Can you work these out from the model? Positions are in its coordinate system, mm. Face numbers are marked on the shaded views. A direction names the side the tool comes from. Coordinates: 2 decimals unless noted, no trailing zeros. Order: outer loops, then holes, each group sorted by start corner. A loop starts at its lowest first (then second) coordinate and runs counter-clockwise, first axis right, second up. Notation, with made-up numbers: (34, -27.5) -> (92, -27.5) arc R18 ccw to (92, -9.5) -> close; hole circle Ø9 at (38.5, 45.5). An arc over 180 degrees is marked (long way). Answer in a Markdown table with one row per item.
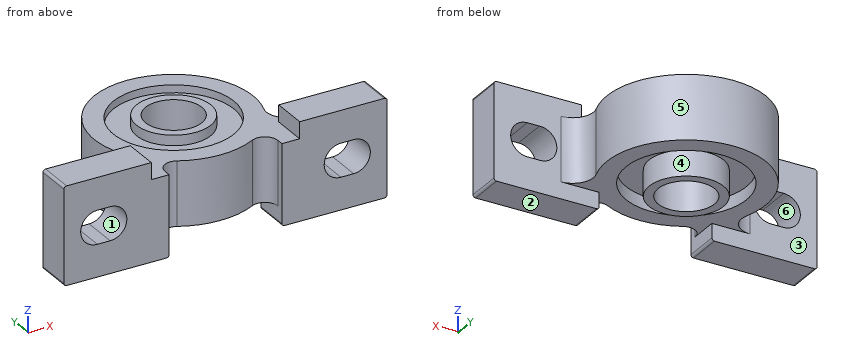
```python
from build123d import *

# Parameters (mm, degrees)
SKETCH_8_R          = 14.5
SKETCH_8_R_2        = 11
EXTRUDE_1_DEPTH     = 31
SKETCH_10_R         = 23.5
SKETCH_10_R_2       = 14.5
EXTRUDE_2_DEPTH     = 17
EXTRUDE_START       = -5
SKETCH_11_R         = 31
SKETCH_11_R_2       = 23.5
EXTRUDE_3_DEPTH     = 25
SKETCH_13_W         = 41
SKETCH_13_H         = 38
EXTRUDE_4_DEPTH     = 14
FILLET_1_R          = 8
FILLET_2_R          = 5
FILLET_3_R          = 5
FILLET_4_R          = 8
FILLET_5_R          = 1
FILLET_6_R          = 1
SKETCH_14_W         = 12.689774382
SKETCH_14_H         = 9.496761799
CUT_EXTRUDE_5_DEPTH = 130.435312029


with BuildPart() as part:
    # Эскиз8 → Вытянуть1 (new body)
    with BuildSketch(Plane.XY):
        with Locations((50, -1.5)):
            Circle(SKETCH_8_R)
        with Locations((50, -1.5)):
            Circle(SKETCH_8_R_2, mode=Mode.SUBTRACT)
    extrude(amount=EXTRUDE_1_DEPTH)

    # Эскиз10 → Вытянуть2 (add)
    with BuildSketch(Plane.XY.offset(10)):
        with Locations((50, -1.5)):
            Circle(SKETCH_10_R)
        with Locations((50, -1.5)):
            Circle(SKETCH_10_R_2, mode=Mode.SUBTRACT)
    extrude(amount=EXTRUDE_2_DEPTH)

    # Эскиз11 → Вытянуть3 (add)
    with BuildSketch(Plane.XY.offset(10).offset(EXTRUDE_START)):
        with Locations((50, -1.5)):
            Circle(SKETCH_11_R)
        with Locations((50, -1.5)):
            Circle(SKETCH_11_R_2, mode=Mode.SUBTRACT)
    extrude(amount=EXTRUDE_3_DEPTH)

    # Эскиз13 → Вытянуть4 (add)
    # profile 1 of 2: a face of its own
    with BuildSketch(Plane(origin=(0, -36, 0), x_dir=(-1, 0, 0), z_dir=(0, 1, 0))):
        with Locations((-7.5, 17.5)):
            Rectangle(SKETCH_13_W, SKETCH_13_H)
        with BuildLine():
            Line((-4.740103958, 23.994802079), (0, 24))
            ThreePointArc((0, 24), (6.5, 17.5), (0, 11))
            Line((0, 11), (-5, 11))
            ThreePointArc((-5, 11), (-11.49870039, 17.629974008), (-4.740103958, 23.994802079))
        make_face(mode=Mode.SUBTRACT)
    # profile 2 of 2: a face of its own
    with BuildSketch(Plane(origin=(0, -36, 0), x_dir=(-1, 0, 0), z_dir=(0, 1, 0))):
        with Locations((-92.5, 17.5)):
            Rectangle(SKETCH_13_W, SKETCH_13_H)
        with BuildLine():
            Line((-95, 11), (-100, 11))
            ThreePointArc((-100, 11), (-106.5, 17.5), (-100, 24))
            Line((-100, 24), (-95.259896042, 23.994802079))
            ThreePointArc((-95.259896042, 23.994802079), (-88.50129961, 17.629974008), (-95, 11))
        make_face(mode=Mode.SUBTRACT)
    extrude(amount=EXTRUDE_4_DEPTH)

    # Скругление1
    fillet_1_edges = [part.edges().sort_by_distance(p)[0] for p in [
        (26.745968092, -22, 17.5),
    ]]
    fillet(fillet_1_edges, radius=FILLET_1_R)

    # Скругление2
    fillet_2_edges = [part.edges().sort_by_distance(p)[0] for p in [
        (28, -23.340329668, 17.5),
    ]]
    fillet(fillet_2_edges, radius=FILLET_2_R)

    # Скругление3
    fillet_3_edges = [part.edges().sort_by_distance(p)[0] for p in [
        (72, -23.340329668, 17.5),
    ]]
    fillet(fillet_3_edges, radius=FILLET_3_R)

    # Скругление4
    fillet_4_edges = [part.edges().sort_by_distance(p)[0] for p in [
        (73.254031908, -22, 17.5),
    ]]
    fillet(fillet_4_edges, radius=FILLET_4_R)

    # Скругление5
    fillet_5_edges = [part.edges().sort_by_distance(p)[0] for p in [
        (28, -29, 36.5),
        (28, -29, -1.5),
        (72, -29, -1.5),
        (72, -29, 36.5),
    ]]
    fillet(fillet_5_edges, radius=FILLET_5_R)

    # Скругление6
    fillet_6_edges = [part.edges().sort_by_distance(p)[0] for p in [
        (-13, -29, -1.5),
        (-13, -29, 36.5),
        (113, -29, 36.5),
        (113, -29, -1.5),
    ]]
    fillet(fillet_6_edges, radius=FILLET_6_R)

    # Эскиз14 → Вытянуть5 (cut, through all)
    with BuildSketch(Plane(origin=(0, -22, 0), x_dir=(1, 0, 0), z_dir=(0, 1, 0))):
        with Locations((27.402364267, -34.7483809)):
            Rectangle(SKETCH_14_W, SKETCH_14_H)
        with Locations((72.597635733, -34.7483809)):
            Rectangle(SKETCH_14_W, SKETCH_14_H)
    extrude(amount=-CUT_EXTRUDE_5_DEPTH, mode=Mode.SUBTRACT)


solid = part.part
```
(1) Suppose I cut it at D-D (z = 17.5). Please give me the cut outline in (x, y), and give its area (3 significant figures).
Response values:
| item | result |
|---|---|
| outline | (-13, -36) -> (-6.5, -36) -> (-6.5, -22) -> (-13, -22) -> close; (11.5, -36) -> (28, -36) -> (28, -33.23) arc R5 cw to (35.36, -28.83) arc R31 ccw to (64.64, -28.83) arc R5 cw to (72, -33.23) -> (72, -36) -> (88.5, -36) -> (88.5, -22) -> (86.94, -22) arc R8 cw to (79.36, -11.44) arc R31 ccw (long way) to (20.64, -11.44) arc R8 cw to (13.06, -22) -> (11.5, -22) -> close; (106.5, -36) -> (113, -36) -> (113, -22) -> (106.5, -22) -> close; hole circle Ø22 at (50, -1.5) |
| area | 3,390 mm2 |
(2) We'd pull the mould along X, two halves only. Please class the marked faces 3, 4, 5 and 6: +X half, -X half, draft (parallel to the pull), parting line (faces both ways), or undercut.
Response values:
| item | result |
|---|---|
| face 3 | draft |
| face 4 | undercut |
| face 5 | parting line |
| face 6 | undercut |
(3) Suppose I cut it at A-A (z = 7). Please give me the cut outline in (x, y), and give its area (3 significant figures).
Response values:
| item | result |
|---|---|
| outline | (-13, -36) -> (28, -36) -> (28, -33.23) arc R5 cw to (35.36, -28.83) arc R31 ccw to (64.64, -28.83) arc R5 cw to (72, -33.23) -> (72, -36) -> (113, -36) -> (113, -22) -> (86.94, -22) arc R8 cw to (79.36, -11.44) arc R31 ccw (long way) to (20.64, -11.44) arc R8 cw to (13.06, -22) -> (-13, -22) -> close; circle Ø29 at (50, -1.5); hole circle Ø47 at (50, -1.5); hole circle Ø22 at (50, -1.5) |
| area | 2,820 mm2 |
(4) Will these pins go through, and if not, where does the flat tip stop? pin 1 Ø5 at (x, y) = (81.5, 1.5) entering from +Z; pin 2 Ø23.5 at (x, y) = (50, 8) entering from -Z; pin 3 Ø4 at (x, y) = (41.5, 15.5) entering from -Z.
Response values:
| item | result |
|---|---|
| pin 1 | z = 30 |
| pin 2 | z = 0 |
| pin 3 | z = 10 |
(5) On a 3-axis mill with a long thin cutter (end or side, diameter ignored), from which of +Z, -Z, +X, -X, +Y, -Y can I reach the whole of each face in a straight line? I mean the marked faces 1 and 2. Say none if no direction works.
Response values:
| item | result |
|---|---|
| face 1 | +Y, -Y |
| face 2 | -Z, +X, -X, +Y, -Y |
(6) Suppose I cut it at B-B (y = -30.5). Count the separate pieces of the cut face and the enclosed holes in it, and give its area (3 significant figures).
Response values:
| item | result |
|---|---|
| separate pieces | 3 |
| enclosed holes | 2 |
| area | 3,220 mm2 |
(7) Suppose I cut it at C-C (x = 50). Please give me the cut outline in (y, z).
Response values:
| item | result |
|---|---|
| outline | (-32.5, 5) -> (-25, 5) -> (-25, 10) -> (-16, 10) -> (-16, 0) -> (-12.5, 0) -> (-12.5, 31) -> (-16, 31) -> (-16, 27) -> (-25, 27) -> (-25, 30) -> (-32.5, 30) -> close; (9.5, 0) -> (13, 0) -> (13, 10) -> (22, 10) -> (22, 5) -> (29.5, 5) -> (29.5, 30) -> (22, 30) -> (22, 27) -> (13, 27) -> (13, 31) -> (9.5, 31) -> close |
(8) I need wall thicknesses on line 1 (Y direction, x = 50, z = 29.1); line 2 (X direction, y = -1, z = 7); line 3 (X direction, y = -27, z = 14). Which ranges of each line are inside material? Lowest first, please. Write a range as [from, to].
Response values:
| item | result |
|---|---|
| line 1 | [-32.5, -25], [-16, -12.5], [9.5, 13], [22, 29.5] |
| line 2 | [19, 26.51], [35.51, 39.01], [60.99, 64.49], [73.49, 81] |
| line 3 | [-13, -5.48], [10.48, 89.52], [105.48, 113] |
